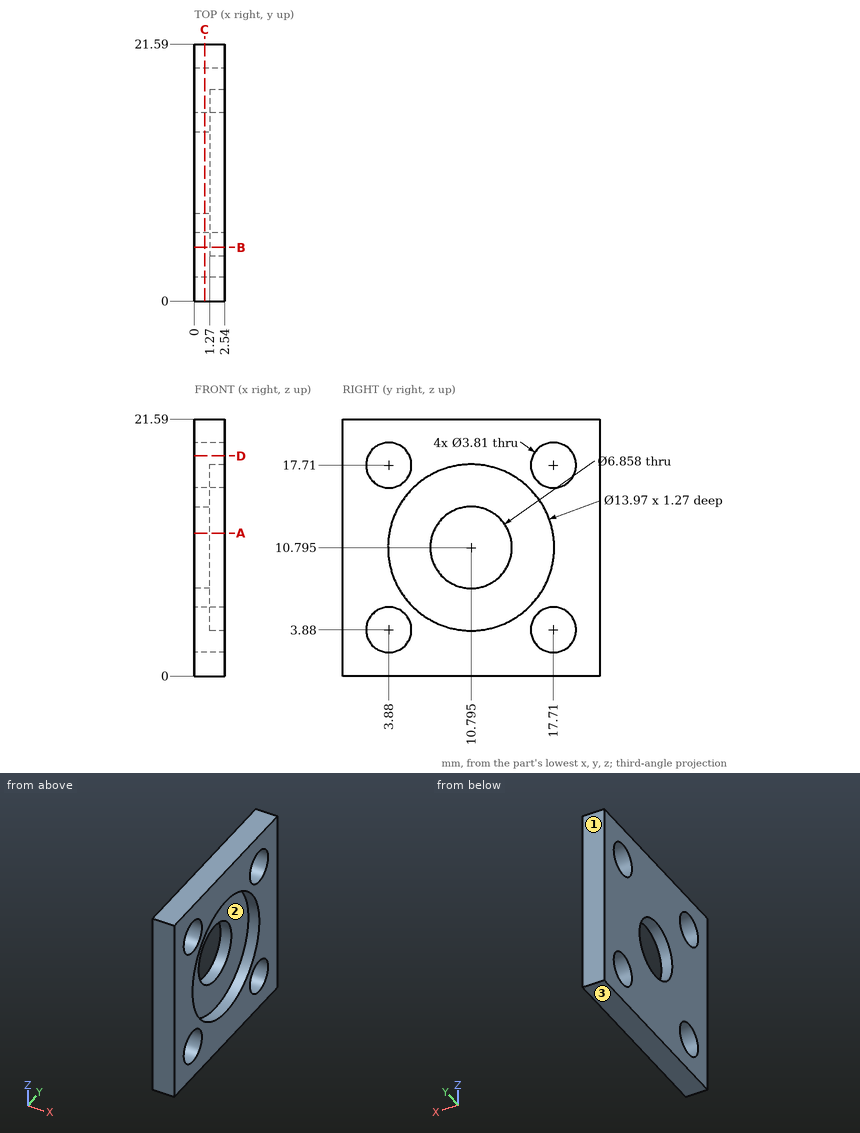
Part print with two shaded views. Sizes in mm from the minimum x, y, z corner. Round coordinates to 2 decimals unless told otherwise and drop trailing zeros. Order: outer loops, then holes, each group sorted by start corner. A loop starts at its lowest first (then second) coordinate and runs counter-clockwise, first axis right, second up. Notation, with made-up numbers: M -37,42.5 L -9,42.5 A6 cw -9,46.5 Z; hole C -38.5,15.25 d10. An arc over 180 degrees is marked long. Put each result on its own line as item: value. Start each with the question number.
1. Slice it at C-C on x = 0.85. List the corners of the cut face in (y, z) (1 decimal), then the cut area to 3 significant figures.
2. Slice it at A-A on z = 12. List the corners of the cut face in (x, y) (1 decimal).
3. Drill centre lines: probe 1 along Y at (x, z) = (2.45, 16.25) (1 decimal); probe 2 along Z at (x, y) = (2, 16.5) (1 decimal); probe 3 along Y at (x, z) = (1.8, 17). Where is each one in solid material? Low to high. Write a range as [from, to].
4. Slice it at B-B on y = 4.5. List the corners of the cut face in (x, z).
5. Slice it at D-D on z = 18.5. List the corners of the cut face in (x, y).
6. Two-plate mould, pull along Y, no slides. Class the marked faces 1, 2 and 3: +Y half, -Y half, draft (parallel to the pull), parting line (faces both ways), or undercut.
Findings:
1. outline: M 0,0 L 21.6,0 L 21.6,21.6 L 0,21.6 Z; hole C 3.9,3.9 d3.8; hole C 3.9,17.7 d3.8; hole C 10.8,10.8 d6.9; hole C 17.7,3.9 d3.8; hole C 17.7,17.7 d3.8
1. area: 384 mm2
2. outline: M 0,0 L 2.5,0 L 2.5,3.9 L 1.3,3.9 L 1.3,7.6 L 0,7.6 Z; M 0,14 L 1.3,14 L 1.3,17.7 L 2.5,17.7 L 2.5,21.6 L 0,21.6 Z
3. probe 1: [0, 2.7], [5.1, 6.4], [15.2, 16.5], [18.9, 21.6]
3. probe 2: [0, 2.4], [5.4, 6.8], [14.8, 16.2], [19.2, 21.6]
3. probe 3: [0, 2.11], [5.65, 7.59], [14, 15.94], [19.48, 21.59]
4. outline: M 0,0 L 2.54,0 L 2.54,2.08 L 0,2.08 Z; M 0,5.68 L 2.54,5.68 L 2.54,7.77 L 1.27,7.77 L 1.27,13.82 L 2.54,13.82 L 2.54,15.91 L 0,15.91 Z; M 0,19.51 L 2.54,19.51 L 2.54,21.59 L 0,21.59 Z
5. outline: M 0,0 L 2.54,0 L 2.54,2.15 L 0,2.15 Z; M 0,5.61 L 2.54,5.61 L 2.54,15.98 L 0,15.98 Z; M 0,19.44 L 2.54,19.44 L 2.54,21.59 L 0,21.59 Z
6. face 1: +Y half
6. face 2: undercut
6. face 3: draft
